```python
from build123d import *

# Parameters (mm, degrees)
SKETCH1_W           = 140
SKETCH1_H           = 165
SKETCH1_R           = 2.125
SKETCH1_R_2         = 7
BOSS_EXTRUDE1_DEPTH = 3.175
SKETCH2_R           = 2.125
CUT_EXTRUDE1_DEPTH  = 109.242000282


with BuildPart() as part:
    # Sketch1 → Boss-Extrude1 (new body)
    with BuildSketch(Plane.XY):
        Rectangle(SKETCH1_W, SKETCH1_H)
        with Locations((0, 71.5)):
            Circle(SKETCH1_R, mode=Mode.SUBTRACT)
        with Locations((25.11473671, 28)):
            Circle(SKETCH1_R, mode=Mode.SUBTRACT)
        with Locations((-25.11473671, 28)):
            Circle(SKETCH1_R, mode=Mode.SUBTRACT)
        with Locations((0, 42.5)):
            Circle(SKETCH1_R_2, mode=Mode.SUBTRACT)
        with Locations((-62, -74.5)):
            Circle(SKETCH1_R, mode=Mode.SUBTRACT)
        with Locations(Location((-38, -74.5, 0), (0, 0, 180))):
            Circle(SKETCH1_R, mode=Mode.SUBTRACT)
        with Locations((-38, -50.5)):
            Circle(SKETCH1_R, mode=Mode.SUBTRACT)
        with Locations(Location((-62, -50.5, 0), (0, 0, 180))):
            Circle(SKETCH1_R, mode=Mode.SUBTRACT)
        with Locations((38, -74.5)):
            Circle(SKETCH1_R, mode=Mode.SUBTRACT)
        with Locations(Location((62, -74.5, 0), (0, 0, 180))):
            Circle(SKETCH1_R, mode=Mode.SUBTRACT)
        with Locations((62, -50.5)):
            Circle(SKETCH1_R, mode=Mode.SUBTRACT)
        with Locations(Location((38, -50.5, 0), (0, 0, 180))):
            Circle(SKETCH1_R, mode=Mode.SUBTRACT)
    extrude(amount=BOSS_EXTRUDE1_DEPTH)

    # Sketch2 → Cut-Extrude1 (cut, through all)
    with BuildSketch(Plane.XY.offset(3.175)):
        with Locations((-62, 74.5)):
            Circle(SKETCH2_R)
        with Locations((-62, 40.5)):
            Circle(SKETCH2_R)
        with Locations((-62, 6.5)):
            Circle(SKETCH2_R)
        with Locations((-62, -27.5)):
            Circle(SKETCH2_R)
        with Locations((-28, 6.5)):
            Circle(SKETCH2_R)
        with Locations((-28, -27.5)):
            Circle(SKETCH2_R)
        with Locations(Location((28, -27.5, 0), (0, 0, 180))):
            Circle(SKETCH2_R)
        with Locations(Location((28, 6.5, 0), (0, 0, 180))):
            Circle(SKETCH2_R)
        with Locations(Location((62, -27.5, 0), (0, 0, 180))):
            Circle(SKETCH2_R)
        with Locations(Location((62, 6.5, 0), (0, 0, 180))):
            Circle(SKETCH2_R)
        with Locations(Location((62, 40.5, 0), (0, 0, 180))):
            Circle(SKETCH2_R)
        with Locations(Location((62, 74.5, 0), (0, 0, 180))):
            Circle(SKETCH2_R)
    extrude(amount=-CUT_EXTRUDE1_DEPTH, mode=Mode.SUBTRACT)


solid = part.part
```
The listing builds one solid part. Answer for the finished solid, in the listing's coordinates (mm). Coordinates: 2 decimals unless noted, no trailing zeros. Loops run counter-clockwise (first coordinate to the right, second up) from the corner with the lowest first, then second, coordinate; pieces in that order, holes last. Notation, with made-up numbers: (36.25, 4) -> (42.25, 4) arc R11 cw to (42.25, 19) -> close; hole circle Ø10 at (-11, 37.25). An arc over 180 degrees is marked (long way). Return JSON: item names as keys, results as strings. Group by question number.
(1) A cutting plane is placed at D-D on y = 40.5. Write down the section's boundary in (x, z) (3 decimals), and give its area (3 significant figures).
(2) Given pin 1 Ø4 at (x, y) = (-28, 6.5) entering from +Z, flat-ended and moving along its own axis, determine where the tip first touches the part or whether it passes through.
(3) Determine the mould class of faces 1 (the flat face through (-1, 1, 0)), 2 (the cylindrical face through (64.123, -27.593, 1.61)) for opening direction X: released by +X, released by -X, zero draft, split by the parting line, or undercut.
(4) Find the intervals of material crossed by probe 1 along Y at (x, z) = (25, 0.1); probe 2 along Y at (x, z) = (0, 1.15) (3 decimals); probe 3 along X at (y, z) = (38, 2.3), in increasing order. Write a range as from..to.
(5) A cutting plane is placed at A-A on y = -74.5. Write down the section's boundary in (x, z) (3 decimals).
(6) A cutting plane is placed at B-B on x = -38. Write down the section's boundary in (y, z) (3 decimals), and give its area (3 significant figures).
(7) A cutting plane is placed at C-C on z = 1.8. Count the separate pieces of the cut face and the enclosed holes in it, and give its area (3 significant figures).
The answers:
{
 "1": {"outline": "(-70, 0) -> (-64.125, 0) -> (-64.125, 3.175) -> (-70, 3.175) -> close; (-59.875, 0) -> (-6.708, 0) -> (-6.708, 3.175) -> (-59.875, 3.175) -> close; (6.708, 0) -> (59.875, 0) -> (59.875, 3.175) -> (6.708, 3.175) -> close; (64.125, 0) -> (70, 0) -> (70, 3.175) -> (64.125, 3.175) -> close", "area": "375 mm^2"},
 "2": {"pin 1": "passes through"},
 "3": {"face 1": "zero draft", "face 2": "undercut"},
 "4": {"probe 1": "y = -82.5..25.88, 30.12..82.5", "probe 2": "y = -82.5..35.5, 49.5..69.375, 73.625..82.5", "probe 3": "x = -70..-5.36, 5.36..70"},
 "5": {"outline": "(-70, 0) -> (-64.125, 0) -> (-64.125, 3.175) -> (-70, 3.175) -> close; (-59.875, 0) -> (-40.125, 0) -> (-40.125, 3.175) -> (-59.875, 3.175) -> close; (-35.875, 0) -> (35.875, 0) -> (35.875, 3.175) -> (-35.875, 3.175) -> close; (40.125, 0) -> (59.875, 0) -> (59.875, 3.175) -> (40.125, 3.175) -> close; (64.125, 0) -> (70, 0) -> (70, 3.175) -> (64.125, 3.175) -> close"},
 "6": {"outline": "(-82.5, 0) -> (-76.625, 0) -> (-76.625, 3.175) -> (-82.5, 3.175) -> close; (-72.375, 0) -> (-52.625, 0) -> (-52.625, 3.175) -> (-72.375, 3.175) -> close; (-48.375, 0) -> (82.5, 0) -> (82.5, 3.175) -> (-48.375, 3.175) -> close", "area": "497 mm^2"},
 "7": {"separate pieces": "1", "enclosed holes": "24", "area": "22,600 mm^2"}
}
